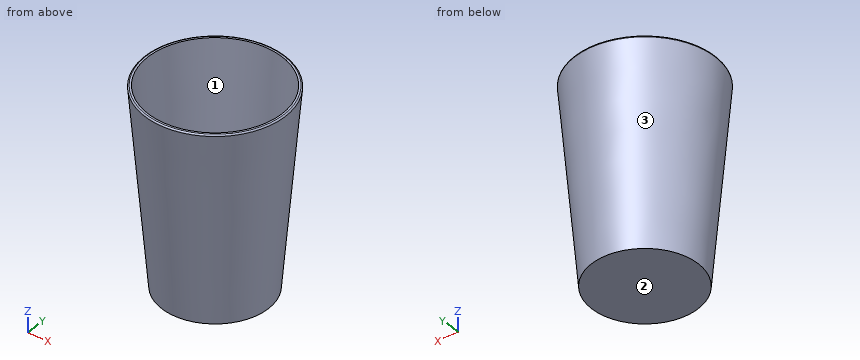
from build123d import *

# Parameters (mm, degrees)
F0_R     = 40.7452616352
F1_DEPTH = 150
F1_TAPER = -5
F2_T     = -2.54
F3_R     = 1


with BuildPart() as f1:
    # F0 (on Top) → F1 (new body)
    with BuildSketch(Plane.XY):
        Circle(F0_R)
    extrude(amount=F1_DEPTH, taper=F1_TAPER)

    # F2
    f2_openings = [f1.faces().sort_by_distance(p)[0] for p in [
        (0, 0, 150),
    ]]
    offset(amount=F2_T, openings=f2_openings, kind=Kind.INTERSECTION)

    # F3
    f3_edges = [f1.edges().sort_by_distance(p)[0] for p in [
        (-53.868561, 0, 150),
    ]]
    fillet(f3_edges, radius=F3_R)


solid = f1.part
Could you check a few things on this model? Use its own coordinates, in mm. Face numbers are marked on the shaded views. Give positions to 0.01 mm unless a question says otherwise; leave off trailing zeros. Order: outer loops, then holes, each group sorted by start corner. A loop starts at its lowest first (then second) coordinate and runs counter-clockwise, first axis right, second up.
1. Suppose I cut it at B-B (z = 72). List the corners of the cut face in (x, y) for me.
2. We'd pull the mould along Y, two halves only. Please class the marked faces 1, 2 and 3: pulls with the +Y half, pulls with the -Y half, needs draft (parallel to the pull), parting line crosses it, or undercut.
3. Suppose I cut it at A-A (x = 0). List the corners of the cut face in (y, z) for me, plus the area to 3 significant figures.
4. Will these pins go through, and if not, where does the flat tip stop? P1, Ø8, axis at x = -28, z = 97, coming from the -Y side; P2, Ø2, axis at x = 8.5, y = -20, coming from the -Z side; P3, Ø5, axis at x = -38.5, z = 105.5, coming from the +Y side; P4, Ø5, axis at x = -33, z = 96.5, coming from the -Y side.
5. I need wall thicknesses on L1, parallel to Y at x = 11.5, z = 87.5; L2, parallel to X at y = -10.5, z = 13; L3, parallel to Z at x = 8, y = -17.5. Which ranges of each line are inside material? Lowest first, please.
6. Suppose I cut it at C-C (z = 44.5). List the corners of the cut face in (x, y) for me, plus the area to 3 significant figures.
Solved:
1. outline: circle Ø94.09 at (0, 0); hole circle Ø88.99 at (0, 0)
2. face 1: undercut
2. face 2: needs draft
2. face 3: parting line crosses it
3. outline: (-53.77, 148.91) - (-40.75, 0) - (40.75, 0) - (53.77, 148.91) arc R1 ccw to (52.78, 150) - (51.32, 150) - (38.42, 2.54) - (-38.42, 2.54) - (-51.32, 150) - (-52.78, 150) arc R1 ccw to start
3. area: 959 mm2
4. P1: stops at y = -43.02
4. P2: stops at z = 0
4. P3: stops at y = 34.68
4. P4: stops at y = -38.61
5. L1: y = -47.01 to -44.39, 44.39 to 47.01
5. L2: x = -40.55 to -37.91, 37.91 to 40.55
5. L3: z = 0 to 2.54
6. outline: circle Ø89.28 at (0, 0); hole circle Ø84.18 at (0, 0)
6. area: 695 mm2
